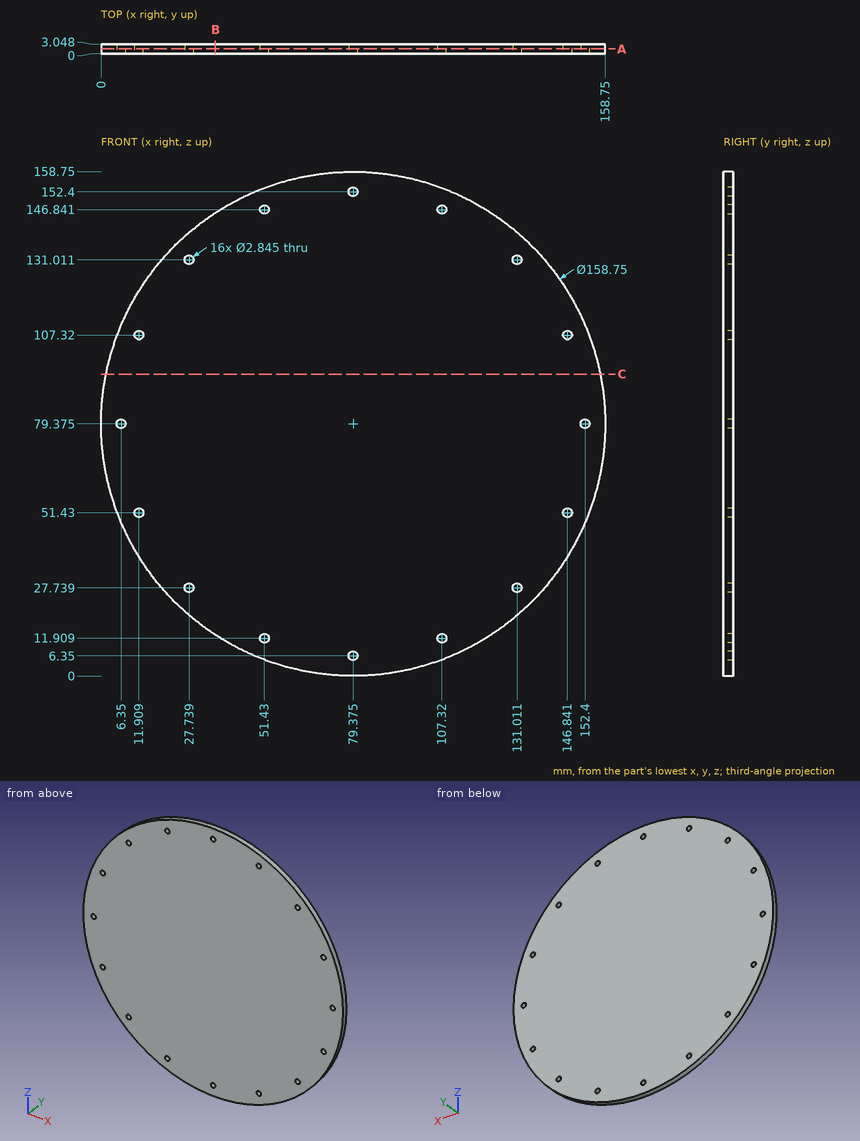
Study the drawing (mm; zero at the part's minimum x, y, z) and answer. Coordinates: 2 decimals unless noted, no trailing zeros. Write each loop counter-clockwise with the first axis right and the second up, starting at its lowest first coordinate (ties: lowest second). Pieces come first, ordered by that corner, then holes. Notation, with made-up numbers: (42, 28.25) -> (47, 28.25) arc R20 ccw to (47, 42.25) -> close; hole circle Ø1 at (21.25, 53). An arc over 180 degrees is marked (long way). Write item = value, one per line.
(1) Section C-C on z = 95 is taken. Write down the section's boundary in (x, y).
From the geometry:
outline = (1.55, 0) -> (157.2, 0) -> (157.2, 3.05) -> (1.55, 3.05) -> close
(2) Straight lines are drawn through the part: L1, parallel to X at y = 0.5, z = 107 (1 decimal); L2, parallel to Z at x = 131, y = 0.4 (1 decimal); L3, parallel to Z at x = 52, y = 1.4 (1 decimal). For each, find the intervals that lie inside material, in ascending order. Write a range as from..to.
From the geometry:
L1 = 5..10.5, 13.3..145.5, 148.2..153.8
L2 = 19.1..26.3, 29.2..129.6, 132.4..139.7
L3 = 4.9..10.6, 13.2..145.5, 148.1..153.9
(3) Section A-A on y = 1.55 is taken. Count the separate pieces of the cut face and the enclosed holes in it, plus the area to 3 significant figures.
From the geometry:
separate_pieces = 1
enclosed_holes = 16
area = 19,700 mm2
(4) Section B-B on x = 36 is taken. Write down the section's boundary in (y, z).
From the geometry:
outline = (0, 12.9) -> (3.05, 12.9) -> (3.05, 145.85) -> (0, 145.85) -> close
(5) Given pin 1 Ø3.5 at (x, z) = (79.375, 152.4) entering from -Y; pin 2 Ø1.5 at (y, z) = (1.5, 131) entering from +X, each flat-ended and moving along its own axis, determine where each tip first touches the part or whether it passes through.
From the geometry:
pin_1 = 0
pin_2 = 140.3
